The listing builds one solid part. Answer for the finished solid, in the listing's coordinates (mm). A direction names the side the tool comes from. Round coordinates to 2 decimals unless told otherwise and drop trailing zeros. Write each loop counter-clockwise with the first axis right and the second up, starting at its lowest first coordinate (ties: lowest second). Pieces come first, ordered by that corner, then holes. Notation, with made-up numbers: (-4.75, 3) - (45.25, 3) arc R16 cw to (45.25, 24) - close; hole circle Ø3 at (42, 57.25). An arc over 180 degrees is marked (long way). Return JSON: item names as keys, results as strings. Group by question number.
(1) Find the intervals of material crossed by line 1 along Z through (x, y) = (29.15, 15); line 2 along Z through (x, y) = (8, 15); line 3 along Y through (x, z) = (15, 20), in increasing order. Write a range as [from, to].
(2) Section A-A, the plane x = 23 is taken. Write down the section's boundary in (y, z).
(3) Section D-D, the plane z = 15 is taken. Give the number of separate pieces and of enclosed holes in the cut face, then the cut area to 3 significant figures.
(4) Each of these flat-tipped pins is pushed along its axis until it touches: pin 1 (15.5 mm diameter, centred on y = 15, z = 15, fed in from -X); pin 2 (9.5 mm diameter, centred on y = 17, z = 12.5, fed in from -X); pin 3 (2 mm diameter, centred on y = 14, z = 4.5, fed in from -X); pin 4 (6 mm diameter, centred on x = 13.5, z = 15.5, fed in from +Y). Where does it stop, or does it pass through?
(5) Section C-C, the plane z = 6 is taken. Write down the section's boundary in (x, y), then the cut area to 3 significant figures.
(6) Which of the six approach directions +Z, -Z, +X, -X, +Y, -Y give full straight-line access (tool end or side, diameter ignored) to faces 1 (the cylindrical face through (10.933, 18.763, 0.114)), 2 (the cylindrical face through (11.774, 7.583, 20.059)), 3 (the cylindrical face through (22.417, 11.774, 20.059))?
(7) Determine the mould class of faces 4 (the flat face through (11, 19, 8)), 5 (the flat face through (12, 3, 12)), 6 (the flat face through (18, 12, 30)), 7 (the flat face through (30, 14.6, 11.6)) for opening direction X: +X half, -X half, draft (parallel to the pull), parting line (faces both ways), or undercut.
```python
from build123d import *

# Parameters (mm, degrees)
BOSS_EXTRUDE1_DEPTH = 30
SKETCH3_R           = 3.2
CUT_EXTRUDE8_DEPTH  = 33
SKETCH5_R           = 3.2
CUT_EXTRUDE5_DEPTH  = 32
CUT_EXTRUDE9_START  = -27
SKETCH8_R           = 6
SKETCH8_R_2         = 3.2
CUT_EXTRUDE9_DEPTH  = 27
CUT_EXTRUDE10_START = -27
SKETCH7_R           = 6
SKETCH7_R_2         = 3.2
CUT_EXTRUDE10_DEPTH = 27
FILLET6_R           = 0.4


with BuildPart() as part:
    # Sketch2 → Boss-Extrude1 (new body)
    with BuildSketch(Plane.XY):
        Polygon((0, 0), (30, 0), (30, 30), (22, 30), (0, 8), align=None)
    extrude(amount=BOSS_EXTRUDE1_DEPTH)

    # Sketch3 → Cut-Extrude8 (cut)
    with BuildSketch(Plane(origin=(30, 0, 0), x_dir=(0, 0, -1), z_dir=(1, 0, 0))):
        with Locations((-15, 15)):
            Circle(SKETCH3_R)
    extrude(amount=-CUT_EXTRUDE8_DEPTH, mode=Mode.SUBTRACT)

    # Sketch5 → Cut-Extrude5 (cut)
    with BuildSketch(Plane.XZ):
        with Locations(Location((15, 15, 0), (0, 0, 270))):
            Circle(SKETCH5_R)
    extrude(amount=-CUT_EXTRUDE5_DEPTH, mode=Mode.SUBTRACT)

    # Sketch8 → Cut-Extrude9 (cut)
    with BuildSketch(Plane.ZY.offset(CUT_EXTRUDE9_START)):
        with Locations(Location((15, 15, 0), (0, 0, 270))):
            Circle(SKETCH8_R)
        with Locations(Location((15, 15, 0), (0, 0, 180))):
            Circle(SKETCH8_R_2, mode=Mode.SUBTRACT)
    extrude(amount=CUT_EXTRUDE9_DEPTH, mode=Mode.SUBTRACT)

    # Sketch7 → Cut-Extrude10 (cut)
    with BuildSketch(Plane(origin=(0, 30, 0), x_dir=(1, 0, 0), z_dir=(0, 1, 0)).offset(CUT_EXTRUDE10_START)):
        with Locations(Location((15, -15, 0), (0, 0, 180))):
            Circle(SKETCH7_R)
        with Locations(Location((15, -15, 0), (0, 0, 90))):
            Circle(SKETCH7_R_2, mode=Mode.SUBTRACT)
    extrude(amount=CUT_EXTRUDE10_DEPTH, mode=Mode.SUBTRACT)

    # Fillet6
    fillet6_edges = [part.edges().sort_by_distance(p)[0] for p in [
        (30, 30, 15),
        (26, 30, 30),
        (30, 15, 30),
        (15, 0, 30),
        (0, 4, 30),
        (0, 0, 15),
        (15, 0, 0),
        (30, 15, 0),
        (26, 30, 0),
        (0, 4, 0),
        (22, 30, 15),
        (11, 19, 30),
        (0, 8, 15),
        (11, 19, 0),
        (5.06442792, 13.06442792, 9.320778158),
        (20.999999992, 28.999999992, 15.00031642),
    ]]
    fillet(fillet6_edges, radius=FILLET6_R)


solid = part.part
```
Working result:
{
 "1": {"line 1": "z = [0, 11.8], [18.2, 30]", "line 2": "z = [0, 9], [21, 30]", "line 3": "y = [0, 3]"},
 "2": {"outline": "(0, 0.4) arc R0.4 ccw to (0.4, 0) - (29.6, 0) arc R0.4 ccw to (30, 0.4) - (30, 29.6) arc R0.4 ccw to (29.6, 30) - (0.4, 30) arc R0.4 ccw to (0, 29.6) - close; hole circle Ø12 at (15, 15)"},
 "3": {"separate pieces": "3", "enclosed holes": "0", "area": "276 mm^2"},
 "4": {"pin 1": "stops at x = 0", "pin 2": "stops at x = 5.89", "pin 3": "stops at x = 5", "pin 4": "stops at y = 3"},
 "5": {"outline": "(0, 0.4) arc R0.4 ccw to (0.4, 0) - (30, 0) - (30, 29.6) arc R0.4 ccw to (29.6, 30) - (22.17, 30) arc R0.4 ccw to (21.88, 29.88) - (0.12, 8.12) arc R0.4 ccw to (0, 7.83) - close", "area": "658 mm^2"},
 "6": {"face 1": "-Z, -X, +Y", "face 2": "+Y", "face 3": "-X"},
 "7": {"face 4": "-X half", "face 5": "undercut", "face 6": "draft", "face 7": "+X half"}
}
